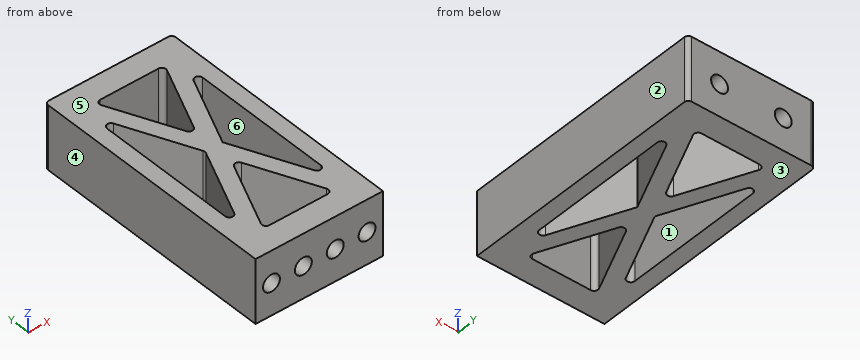
Autodesk Inventor part; units mm, degrees
ref_plane "YZ Plane" through (0, 0, 0) normal (1, 0, 0) x (0, 1, 0)
ref_plane "XZ Plane" through (0, 0, 0) normal (0, 1, 0) x (-1, 0, 0)
ref_plane "XY Plane" through (0, 0, 0) normal (0, 0, 1) x (1, 0, 0)
sketch "Sketch1" plane through (0, 0, 0) normal (0, 1, 0) x (-1, 0, 0)
  line L0 (25.4, 12.7) -> (-25.4, 12.7)
  line L1 (-25.4, 12.7) -> (-25.4, -12.7)
  line L2 (-25.4, -12.7) -> (25.4, -12.7)
  line L3 (25.4, -12.7) -> (25.4, 12.7)
  line L4 (25.4, 12.7) -> (-25.4, -12.7) construction
  line L5 (-25.4, 12.7) -> (25.4, -12.7) construction
  point P0 (0, 0)
  dimension "d0" = 50.8
  dimension "d1" = 25.4
extrude "Extrusion1" add sketch "Sketch1" along normal mid plane 99.06
sketch "Sketch2" plane through (-25.4, 49.53, 12.7) normal (0, 0, 1) x (1, 0, 0)
  line L0 (50.8, -99.06) -> (0, -99.06) construction
  line L1 (0, -99.06) -> (0, 0) construction
  line L2 (0, 0) -> (50.8, 0) construction
  line L3 (50.8, 0) -> (50.8, -99.06) construction
  line L4 (44.45, -6.35) -> (6.35, -6.35) construction
  line L5 (6.35, -6.35) -> (6.35, -92.71) construction
  line L6 (6.35, -92.71) -> (44.45, -92.71) construction
  line L7 (44.45, -92.71) -> (44.45, -6.35) construction
  line L8 (6.35, -6.35) -> (44.45, -92.71) construction
  line L9 (6.35, -92.71) -> (44.45, -6.35) construction
  line L10 (6.35, -14.2159) -> (40.9797, -92.71) construction
  line L11 (44.45, -84.8441) -> (9.8203, -6.35) construction
  line L12 (40.9797, -6.35) -> (6.35, -84.8441) construction
  line L13 (9.8203, -92.71) -> (44.45, -14.2159) construction
  line L14 (0, -99.06) -> (0, 0) construction
  line L15 (0, -89.281) -> (50.8, -89.281) construction
  line L16 (50.8, -99.06) -> (50.8, 0) construction
  line L17 (25.4, -57.3959) -> (11.3331, -89.281)
  line L18 (11.3331, -89.281) -> (39.4669, -89.281)
  line L19 (39.4669, -89.281) -> (25.4, -57.3959)
  line L20 (28.8703, -49.53) -> (44.45, -84.8441)
  line L21 (44.45, -84.8441) -> (44.45, -14.2159)
  line L22 (44.45, -14.2159) -> (28.8703, -49.53)
  line L23 (9.8203, -6.35) -> (25.4, -41.6641)
  line L24 (9.8092, -6.35) -> (40.9797, -6.35) construction
  line L25 (40.9797, -6.35) -> (25.4, -41.6641)
  line L26 (6.35, -14.2159) -> (6.35, -84.8441)
  line L27 (6.35, -84.8441) -> (21.9297, -49.53)
  line L28 (21.9297, -49.53) -> (6.35, -14.2159)
  line L29 (0, -9.779) -> (50.8, -9.779) construction
  line L30 (11.3331, -9.779) -> (39.4669, -9.779)
  point P0 (25.4, -49.53)
  point P1 (9.8203, -6.35)
  dimension "d4" = 6.35
  dimension "d5" = 3.175
  dimension "d6" = 3.175
  dimension "d7" = 3.175
  dimension "d8" = 3.175
  dimension "d9" = 9.779
  dimension "d23" = 9.779
extrude "Extrusion2" cut sketch "Sketch2" against normal through all
fillet "Fillet1" radius 1.5875 13 edges at (-14.0669, -39.751, 0) (-19.05, -35.3141, 0) (14.0669, -39.751, 0) (19.05, -35.3141, 0) (0, 7.8659, 0) (-3.4703, 0, 0) (-19.05, 35.3141, 0) (19.05, 35.3141, 0) (0, -7.8659, 0) (25.4, 49.53, 0) (-25.4, 49.53, 0) (-14.0669, 39.751, 0) (14.0669, 39.751, 0)
sketch "Sketch3" plane through (0, -49.53, 0) normal (0, -1, 0) x (1, 0, 0)
  line L0 (-25.4, 12.7) -> (25.4, 12.7) construction
  line L1 (25.4, 12.7) -> (25.4, -12.7) construction
  line L2 (25.4, -12.7) -> (-25.4, -12.7) construction
  line L3 (-25.4, -12.7) -> (-25.4, 12.7) construction
  line L4 (-6.35, 0) -> (6.35, 0) construction
  point P0 (0, 0)
  point P1 (0, 0)
  point P2 (-19.05, 0)
  point P3 (19.05, 0)
  dimension "d12" = 12.7
  dimension "d13" = 12.7
  dimension "d14" = 12.7
hole "Hole1" at (-6.35, -49.53, 0) at (6.35, -49.53, 0) at (-19.05, -49.53, 0) at (19.05, -49.53, 0) direction (0, 1, 0) diameter 6.75 depth 9.525
sketch "Sketch4" plane through (0, 49.53, 0) normal (0, 1, 0) x (1, 0, 0)
  line L0 (-12.7, 0) -> (12.7, 0) construction
  point P0 (0, 0)
  point P1 (0, 0)
  dimension "d24" = 25.4
hole "Hole2" at (-12.7, 49.53, 0) at (12.7, 49.53, 0) direction (0, -1, 0) diameter 6.75 depth 9.525
equation "\"d6\" = d5"
equation "\"d7\" = d5"
equation "\"d8\" = d7"
equation "\"d23\" = d9"
properties part number "DB1-024" material "ABS Plastic"
Part model, mm, in its own coordinate system. Face numbers are marked on the shaded views. A direction names the side the tool comes from. Give positions to 0.01 mm unless a question says otherwise; leave off trailing zeros. Loops run counter-clockwise (first coordinate to the right, second up) from the corner with the lowest first, then second, coordinate; pieces in that order, holes last.
(1) Drill centre lines: line 1 along X through (y, z) = (-43, 0) (3 decimals); line 2 along X through (y, z) = (47, 0) (3 decimals); line 3 along Z through (x, y) = (-6, -44). Where is each one in solid material? Low to high.
Return value:
line 1: x = -25.4 to -22.425, -15.675 to -9.725, -2.975 to 2.975, 9.725 to 15.675, 22.425 to 25.4
line 2: x = -25.4 to -16.075, -9.325 to 9.325, 16.075 to 25.4
line 3: z = -12.7 to -3.36, 3.36 to 12.7
(2) Pull direction X, two halves, no side cores. Call the marked faces 1, 2, 3 and 4: pulls with the +X half, pulls with the -X half, needs draft (parallel to the pull), parting line crosses it, or undercut.
Return value:
face 1: undercut
face 2: pulls with the +X half
face 3: needs draft
face 4: pulls with the -X half
(3) Band-saw the part on C-C (z = 0). Count the separate pieces of the cut face and the enclosed holes in it, and give its area (3 significant figures).
Return value:
separate pieces: 1
enclosed holes: 4
area: 2,690 mm2
(4) 3-axis set-ups, long thin cutter, end or side, ignore diameter. For the marked faces 5 and 6: which of +Z, -Z, +X, -X, +Y, -Y reach the whole face in a straight line?
Return value:
face 5: +Z, +X, -X, +Y, -Y
face 6: +Z, -Z
(5) Band-saw the part on A-A (y = -17). Write the cut outline in (x, z).
Return value:
outline: (-25.4, -12.7) - (-19.05, -12.7) - (-19.05, 12.7) - (-25.4, 12.7) - close; (-10.97, -12.7) - (-4.03, -12.7) - (-4.03, 12.7) - (-10.97, 12.7) - close; (4.03, -12.7) - (10.97, -12.7) - (10.97, 12.7) - (4.03, 12.7) - close; (19.05, -12.7) - (25.4, -12.7) - (25.4, 12.7) - (19.05, 12.7) - close
(6) Band-saw the part on B-B (x = -6.35). Write the cut outline in (y, z) (3 decimals), and give its area (3 significant figures).
Return value:
outline: (-49.53, -12.7) - (-39.751, -12.7) - (-39.751, 12.7) - (-49.53, 12.7) - (-49.53, 3.375) - (-40.005, 3.375) - (-40.005, -3.375) - (-49.53, -3.375) - close; (-22.259, -12.7) - (-6.527, -12.7) - (-6.527, 12.7) - (-22.259, 12.7) - close; (6.527, -12.7) - (22.259, -12.7) - (22.259, 12.7) - (6.527, 12.7) - close; (39.751, -12.7) - (49.53, -12.7) - (49.53, 12.7) - (39.751, 12.7) - close
area: 1,230 mm2
(7) Pin check, flat tips, straight feed: pin 1 (3.5 mm diameter, centred on x = -12.5, z = 0.5, fed in from +Y) (3 decimals); pin 2 (5.5 mm diameter, centred on x = -6.5, z = 0, fed in from -Y) (3 decimals). Stop position of each tip, or through.
Return value:
pin 1: stops at y = 40.005
pin 2: stops at y = -40.005
